```python
from build123d import *

# Parameters (mm, degrees)
SKETCH_1_W      = 132
SKETCH_1_H      = 40.05
SKETCH_1_R      = 1.6
SKETCH_1_W_2    = 21.2
SKETCH_1_H_2    = 2.6
SKETCH_1_W_3    = 42
EXTRUDE_1_DEPTH = 3
FILLET_1_R      = 5
FILLET_2_R      = 5
FILLET_3_R      = 0.5


with BuildPart() as part:
    # 草图1 → 凸台-拉伸1 (new body)
    with BuildSketch(Plane(origin=(0, 0, 0), x_dir=(1, 0, 0), z_dir=(0, 1, 0))):
        with Locations((-40.850806452, 4.522983871)):
            Rectangle(SKETCH_1_W, SKETCH_1_H)
        with Locations((18.649193548, 19.647983871)):
            Circle(SKETCH_1_R, mode=Mode.SUBTRACT)
        with Locations((18.649193548, -10.152016129)):
            Circle(SKETCH_1_R, mode=Mode.SUBTRACT)
        with Locations((-5.250806452, 19.647983871)):
            Circle(SKETCH_1_R, mode=Mode.SUBTRACT)
        with Locations((-5.250806452, -10.152016129)):
            Circle(SKETCH_1_R, mode=Mode.SUBTRACT)
        with Locations((-100.350806452, -10.152016129)):
            Circle(SKETCH_1_R, mode=Mode.SUBTRACT)
        with Locations((-76.450806452, -10.152016129)):
            Circle(SKETCH_1_R, mode=Mode.SUBTRACT)
        with Locations((-100.350806452, 19.647983871)):
            Circle(SKETCH_1_R, mode=Mode.SUBTRACT)
        with Locations((-76.450806452, 19.647983871)):
            Circle(SKETCH_1_R, mode=Mode.SUBTRACT)
        with Locations((-38.749865004, 8.922983871)):
            Circle(SKETCH_1_R, mode=Mode.SUBTRACT)
        with Locations((-23.050806452, 9.094915776)):
            Circle(SKETCH_1_R, mode=Mode.SUBTRACT)
        with Locations((-51.250806452, 12.122983871)):
            Rectangle(SKETCH_1_W_2, SKETCH_1_H_2, mode=Mode.SUBTRACT)
        with Locations((-40.850806452, -3.077016129)):
            Rectangle(SKETCH_1_W_3, SKETCH_1_H_2, mode=Mode.SUBTRACT)
    extrude(amount=EXTRUDE_1_DEPTH)

    # 圆角1
    fillet_1_edges = [part.edges().sort_by_distance(p)[0] for p in [
        (25.149193548, 1.5, -24.547983871),
    ]]
    fillet(fillet_1_edges, radius=FILLET_1_R)

    # 圆角2
    fillet_2_edges = [part.edges().sort_by_distance(p)[0] for p in [
        (25.149193548, 1.5, 15.502016129),
        (-106.850806452, 1.5, 15.502016129),
        (-106.850806452, 1.5, -24.547983871),
    ]]
    fillet(fillet_2_edges, radius=FILLET_2_R)

    # 圆角3
    fillet_3_edges = [part.edges().sort_by_distance(p)[0] for p in [
        (-40.650806452, 1.5, -10.822983871),
        (-40.650806452, 1.5, -13.422983871),
        (-61.850806452, 1.5, -13.422983871),
        (-61.850806452, 1.5, -10.822983871),
        (-19.850806452, 1.5, 4.377016129),
        (-19.850806452, 1.5, 1.777016129),
        (-61.850806452, 1.5, 1.777016129),
        (-61.850806452, 1.5, 4.377016129),
    ]]
    fillet(fillet_3_edges, radius=FILLET_3_R)


solid = part.part
```
Read the model definition and answer for the solid it produces. Units are mm, in the model's axes. A direction names the side the tool comes from. Give positions to 0.01 mm unless a question says otherwise; leave off trailing zeros. Order: outer loops, then holes, each group sorted by start corner. A loop starts at its lowest first (then second) coordinate and runs counter-clockwise, first axis right, second up. Notation, with made-up numbers: (-24.5, 68.25) -> (24.5, 68.25) arc R26 ccw to (24.5, 96.25) -> close; hole circle Ø7 at (83.5, 44). An arc over 180 degrees is marked (long way). One line per item, written item: value. Start each with the question number.
(1) For a pull along Z with two mould halves and no side action, classify faces 3 (the cylindrical face through (-74.925, 1.479, -20.129)), 4 (the cylindrical face through (-105.425, 1.521, 13.998)), 5 (the cylindrical face through (23.65, 1.52, -23.12)) as released by +Z, released by -Z, zero draft, split by the parting line, or undercut.
(2) The part is cut by section B-B (y = 1.75). State how many separate pieces and enclosed holes the cut face has, and give its area (3 significant figures).
(3) A tool of negligible diameter and unlimited length cuts with its end or side. For faces 1 (the flat face through (-51, 1, -13.423)), 2 (the flat face through (-106.851, 1, -4)), from which of +Z, -Z, +X, -X, +Y, -Y can it reach the whole face along a straight path? Write none if from no direction.
(4) Straight lines are drawn through the part: L1, parallel to Z at x = -44, y = 2.3; L2, parallel to X at y = 1.25, z = -21; L3, parallel to X at y = 2.1, z = 9. For each, find the intervals that lie inside material, in ascending order.
(5) A flat-ended cylindrical pin translates along its axis: P1, Ø2.5, axis at x = -5.25, z = 10.15, coming from the +Y side. Find the tip coordinate at first contact, or state that the pin passes through.
(6) The part is cut by section A-A (x = -29.5). Determine the outline of the cut face in (y, z).
Taken from the geometry:
1. face 3: undercut
1. face 4: released by +Z
1. face 5: released by -Z
2. separate pieces: 1
2. enclosed holes: 12
2. area: 5,020 mm^2
3. face 1: +Y, -Y
3. face 2: +Z, -Z, -X, +Y, -Y
4. L1: -24.55 to -13.42, -10.82 to 1.78, 4.38 to 15.5
4. L2: -106.64 to -101.21, -99.5 to -77.31, -75.6 to -6.11, -4.4 to 17.79, 19.5 to 24.93
4. L3: -106.85 to -101.46, -99.24 to -77.56, -75.34 to -6.36, -4.14 to 17.54, 19.76 to 25.15
5. P1: through
6. outline: (0, -24.55) -> (3, -24.55) -> (3, 1.78) -> (0, 1.78) -> close; (0, 4.38) -> (3, 4.38) -> (3, 15.5) -> (0, 15.5) -> close
